Check sheet for the modelled part. Datum: model origin and axes. Units: mm. A direction names the side the tool comes from. Round coordinates to 2 decimals unless told otherwise and drop trailing zeros. Order: outer loops, then holes, each group sorted by start corner. A loop starts at its lowest first (then second) coordinate and runs counter-clockwise, first axis right, second up.
Q1. Cross-section at D-D on x = -5.75. Record the cut outline in (y, z).
Q2. Scan lines: probe 1 along X at (y, z) = (3.25, 2.63) (3 decimals); probe 2 along X at (y, z) = (3.25, 6.25); probe 3 along Z at (x, y) = (3.75, 0.5). Record each from-to range of solid material in increasing order.
Q3. Cross-section at A-A on z = 2.63. Record the cut outline in (x, y) (3 decimals).
Q4. Mould release check, pull along Z, two halves, no side actions. Record for faces 1 (the flat face through (0, 6.3, 0)), 2 (the cylindrical face through (8.2, 3.14, 7.96)): +Z half, -Z half, draft (parallel to the pull), parting line (faces both ways), or undercut.
Q5. Depth check by flat-ended pin: P1, Ø3, axis at x = 4.5, y = 4.5, coming from the -Z side; P2, Ø3.5, axis at y = 2.5, z = 7.5, coming from the +X side; P3, Ø0.7, axis at x = 8.5, z = 6.5, coming from the -Y side; P4, Ø1.6, axis at x = -2, z = -8.5, coming from the -Y side. Enter the tip coordinate at first touch or a pass-through.
Q6. Set-up check for faces 3 (the flat face through (-8.4, 3, 6)), 4 (the flat face through (2.1, 3, 6)), 5 (the flat face through (9.9, 3, 0)), 6 (the flat face through (-9.9, 3, 0)), 7 (the flat face through (8.5, 3, 6)): record each of +Z, -Z, +X, -X, +Y, -Y from which the full face is reachable in a straight line by a thin tool's end or side.
Q7. Cross-section at B-B on x = 7.5. Record the cut outline in (y, z).
Q8. Cross-section at C-C on z = 7. Record the cut outline in (x, y), then the cut area to 3 significant figures.
from build123d import *

# Parameters (mm, degrees)
SKETCH1_W           = 19.8
SKETCH1_H           = 9.66
MAINBODY_DEPTH      = 6.3
SKETCH2_R           = 1.225
MOUNTINGHOLES_DEPTH = 13.689716309
SKETCH3_W           = 0.6
SKETCH3_H           = 3.2
BOSS_EXTRUDE2_DEPTH = 3.5
SKETCH4_R           = 0.8
CUT_EXTRUDE2_DEPTH  = 22.157478583
SKETCH5_R           = 1.25
BUMPSWITCH_DEPTH    = 2
EXTRUDE_THIN1_DEPTH = 2


with BuildPart() as part:
    # Sketch1 → MainBody (new body)
    with BuildSketch(Plane(origin=(0, 0, 0), x_dir=(1, 0, 0), z_dir=(0, 1, 0))):
        Rectangle(SKETCH1_W, SKETCH1_H)
    extrude(amount=MAINBODY_DEPTH)

    # Sketch2 → MountingHoles (cut, through all)
    with BuildSketch(Plane(origin=(0, 6.3, 0), x_dir=(1, 0, 0), z_dir=(0, 1, 0))):
        with Locations(Location((-4.75, -2.63, 0), (0, 0, 270))):
            Circle(SKETCH2_R)
        with Locations(Location((4.8, -2.63, 0), (0, 0, 270))):
            Circle(SKETCH2_R)
    extrude(amount=-MOUNTINGHOLES_DEPTH, mode=Mode.SUBTRACT)

    # Sketch3 → Boss-Extrude2 (add)
    with BuildSketch(Plane.XY.offset(4.83)):
        with Locations((-8.1, 3.1)):
            Rectangle(SKETCH3_W, SKETCH3_H)
        with Locations((1.8, 3.1)):
            Rectangle(SKETCH3_W, SKETCH3_H)
        with Locations((8.2, 3.1)):
            Rectangle(SKETCH3_W, SKETCH3_H)
    extrude(amount=BOSS_EXTRUDE2_DEPTH)

    # Sketch4 → Cut-Extrude2 (cut, through all)
    with BuildSketch(Plane(origin=(8.5, 0, 0), x_dir=(0, 0, -1), z_dir=(1, 0, 0))):
        with Locations((-7.162962761, 3.1)):
            Circle(SKETCH4_R)
    extrude(amount=-CUT_EXTRUDE2_DEPTH, mode=Mode.SUBTRACT)

    # Sketch5 → BumpSwitch (add, symmetric)
    with BuildSketch(Plane(origin=(0, 3.15, 0), x_dir=(1, 0, 0), z_dir=(0, 1, 0))):
        with Locations((-2.9, 4.83)):
            Circle(SKETCH5_R)
    extrude(amount=BUMPSWITCH_DEPTH, both=True)

    # Sketch6 → Extrude-Thin1 (add, symmetric)
    with BuildSketch(Plane(origin=(0, 3.15, 0), x_dir=(1, 0, 0), z_dir=(0, 1, 0))):
        with BuildLine():
            Line((-7.9, 4.222056191), (-7.9, 4.83))
            ThreePointArc((-7.9, 4.83), (-7.753756221, 5.211453805), (-7.408601461, 5.43))
            Line((-7.408601461, 5.43), (7.80720966, 9.223727798))
            ThreePointArc((7.80720966, 9.223727798), (8.52542957, 10.181011183), (9.647220295, 9.764097659))
            Line((9.647220295, 9.764097659), (9.56321899, 9.709841039))
            ThreePointArc((9.56321899, 9.709841039), (8.516809587, 10.073393654), (7.910350182, 9.146382256))
            Line((7.910350182, 9.146382256), (-7.384409271, 5.332970427))
            ThreePointArc((-7.384409271, 5.332970427), (-7.675692454, 5.148943939), (-7.8, 4.827604127))
            Line((-7.8, 4.827604127), (-7.8, 4.222056191))
            Line((-7.8, 4.222056191), (-7.9, 4.222056191))
        make_face()
    extrude(amount=EXTRUDE_THIN1_DEPTH, both=True)


solid = part.part
Results found:
1. outline: (0, -4.83) - (6.3, -4.83) - (6.3, 1.92) - (0, 1.92) - close; (0, 3.34) - (6.3, 3.34) - (6.3, 4.83) - (0, 4.83) - close; (1.15, -5.84) - (5.15, -5.84) - (5.15, -5.74) - (1.15, -5.74) - close
2. probe 1: x = -9.9 to -5.975, -3.525 to 3.575, 6.025 to 9.9
2. probe 2: x = -8.4 to -7.8, 1.5 to 2.1, 7.9 to 8.5
2. probe 3: z = -4.83 to 2, 3.26 to 4.83
3. outline: (-9.9, 0) - (-5.975, 0) - (-5.975, 6.3) - (-9.9, 6.3) - close; (-3.525, 0) - (3.575, 0) - (3.575, 6.3) - (-3.525, 6.3) - close; (6.025, 0) - (9.9, 0) - (9.9, 6.3) - (6.025, 6.3) - close
4. face 1: draft
4. face 2: undercut
5. P1: stops at z = -8.77
5. P2: stops at x = 8.5
5. P3: stops at y = 1.5
5. P4: passes through
6. face 3: +Z, -X, +Y, -Y
6. face 4: +Z, +Y, -Y
6. face 5: +Z, -Z, +X, +Y, -Y
6. face 6: +Z, -Z, -X, +Y, -Y
6. face 7: +Z, +X, +Y, -Y
7. outline: (0, -4.83) - (6.3, -4.83) - (6.3, 4.83) - (0, 4.83) - close; (1.15, -9.15) - (5.15, -9.15) - (5.15, -9.04) - (1.15, -9.04) - close
8. outline: (-8.4, 1.5) - (-7.8, 1.5) - (-7.8, 2.32) - (-8.4, 2.32) - close; (-8.4, 3.88) - (-7.8, 3.88) - (-7.8, 4.7) - (-8.4, 4.7) - close; (1.5, 1.5) - (2.1, 1.5) - (2.1, 2.32) - (1.5, 2.32) - close; (1.5, 3.88) - (2.1, 3.88) - (2.1, 4.7) - (1.5, 4.7) - close; (7.9, 1.5) - (8.5, 1.5) - (8.5, 2.32) - (7.9, 2.32) - close; (7.9, 3.88) - (8.5, 3.88) - (8.5, 4.7) - (7.9, 4.7) - close
8. area: 2.94 mm2
